from build123d import *

# Parameters (mm, degrees)
SKETCH1_R           = 95
BOSS_EXTRUDE1_DEPTH = 27
SKETCH2_R           = 42.5
CUT_EXTRUDE1_DEPTH  = 138.03649149
SKETCH3_R           = 1.973562568
CUT_EXTRUDE2_DEPTH  = 18.588547
CIRPATTERN1_START   = 8.4114533
CIRPATTERN1_DEPTH   = 18.5885467


# Read off the part's stored shape, not the designer's step: CirPattern1
with BuildPart() as part:
    # Sketch1 → Boss-Extrude1 (new body)
    with BuildSketch(Plane(origin=(0, 0, 0), x_dir=(1, 0, 0), z_dir=(0, 1, 0))):
        with Locations(Location((0, 0, 0), (0, 0, 270))):
            Circle(SKETCH1_R)
    extrude(amount=BOSS_EXTRUDE1_DEPTH)

    # Sketch2 → Cut-Extrude1 (cut, through all)
    with BuildSketch(Plane(origin=(0, 0, 0), x_dir=(1, 0, 0), z_dir=(0, 1, 0))):
        with Locations(Location((0, 0, 0), (0, 0, 270))):
            Circle(SKETCH2_R)
    extrude(amount=CUT_EXTRUDE1_DEPTH, mode=Mode.SUBTRACT)

    # Sketch3 → Cut-Extrude2 (cut)
    with BuildSketch(Plane(origin=(0, 27, 0), x_dir=(1, 0, 0), z_dir=(0, 1, 0))):
        with Locations((-40.882315231, 0)):
            Circle(SKETCH3_R)
    extrude(amount=-CUT_EXTRUDE2_DEPTH, mode=Mode.SUBTRACT)

    # CirPattern1 outline → CirPattern1 (cut)
    with BuildSketch(Plane(origin=(0, 0, 0), x_dir=(1, 0, 0), z_dir=(0, 1, 0)).offset(CIRPATTERN1_START)):
        with BuildLine():
            ThreePointArc((-1.152550318, 42.484369217), (0, 42.5), (1.152550318, 42.484369217))
            ThreePointArc((1.152550318, 42.484369217), (0, 42.855877799), (-1.152550318, 42.484369217))
        make_face()
        with BuildLine():
            ThreePointArc((42.484369217, -1.152550318), (42.855877799, 0), (42.484369217, 1.152550318))
            ThreePointArc((42.484369217, 1.152550318), (42.5, 0), (42.484369217, -1.152550318))
        make_face()
        with BuildLine():
            ThreePointArc((1.152550318, -42.484369217), (0, -42.5), (-1.152550318, -42.484369217))
            ThreePointArc((-1.152550318, -42.484369217), (0, -42.855877799), (1.152550318, -42.484369217))
        make_face()
    extrude(amount=CIRPATTERN1_DEPTH, mode=Mode.SUBTRACT)


solid = part.part
Work out the finished part from the listing and answer in its coordinate system (mm). Coordinates: 2 decimals unless noted, no trailing zeros. Write each loop counter-clockwise with the first axis right and the second up, starting at its lowest first coordinate (ties: lowest second). Pieces come first, ordered by that corner, then holes.
1. Consider line 1 along X through (y, z) = (9.5, 0); line 2 along Z through (x, y) = (2, 14); line 3 along X through (y, z) = (8.25, 0). Determine where each line is inside the solid, lowest interval first.
Results list:
line 1: x = -95 to -42.86, 42.86 to 95
line 2: z = -94.98 to -42.45, 42.45 to 94.98
line 3: x = -95 to -42.5, 42.5 to 95
2. For a pull along Z with two mould halves and no side action, classify faces 1 (the cylindrical face through (12.766, 13.311, 40.537)), 2 (the flat face through (-20, 27, 41)), 3 (the cylindrical face through (-92.74, 13.31, -20.59)) as +Z half, -Z half, draft (parallel to the pull), parting line (faces both ways), or undercut.
Results list:
face 1: undercut
face 2: draft
face 3: parting line
3. The part is cut by section D-D, the plane x = 66. Write down the section's boundary in (y, z), and give its area (3 significant figures).
Results list:
outline: (0, -68.33) - (27, -68.33) - (27, 68.33) - (0, 68.33) - close
area: 3,690 mm2
4. Flat-ended cylindrical pins translate along their axes: pin 1 (4 mm diameter, centred on x = 59, y = 17.5, fed in from +Z); pin 2 (3 mm diameter, centred on x = -9.5, y = 12, fed in from -Z); pin 3 (10 mm diameter, centred on y = 12.5, z = 12, fed in from +X). Find the tip coordinate at first contact, or state that the pin passes through.
Results list:
pin 1: stops at z = 76
pin 2: stops at z = -94.66
pin 3: stops at x = 94.74
5. The part is cut by section A-A, the plane x = -15.5. Write down the section's boundary in (y, z), and give its area (3 significant figures).
Results list:
outline: (0, -93.73) - (27, -93.73) - (27, -39.57) - (0, -39.57) - close; (0, 39.57) - (27, 39.57) - (27, 93.73) - (0, 93.73) - close
area: 2,920 mm2
6. The part is cut by section B-B, the plane y = 11. Write down the section's boundary in (x, z), and give its area (3 significant figures).
Results list:
outline: circle Ø190 at (0, 0); hole (-42.48, -1.15) arc R42.5 ccw to (-1.15, -42.48) arc R1.97 ccw to (1.15, -42.48) arc R42.5 ccw to (42.48, -1.15) arc R1.97 ccw to (42.48, 1.15) arc R42.5 ccw to (1.15, 42.48) arc R1.97 ccw to (-1.15, 42.48) arc R42.5 ccw to (-42.48, 1.15) arc R1.97 ccw to start
area: 22,700 mm2
7. The part is cut by section C-C, the plane z = 38. Write down the section's boundary in (x, y), and give its area (3 significant figures).
Results list:
outline: (-87.07, 0) - (-19.03, 0) - (-19.03, 27) - (-87.07, 27) - close; (19.03, 0) - (87.07, 0) - (87.07, 27) - (19.03, 27) - close
area: 3,670 mm2
